Design review of the part built by this model. Coordinates are the model's own, in mm. Face numbers are marked on the shaded views. A direction names the side the tool comes from. Coordinates: 2 decimals unless noted, no trailing zeros. Write each loop counter-clockwise with the first axis right and the second up, starting at its lowest first coordinate (ties: lowest second). Pieces come first, ordered by that corner, then holes.
Q1. Take a section at B-B (z = 0.6). Give the boundary of the cut face in (x, y), and give its area (3 significant figures).
Q2. Mouldability with a two-part tool opening along X and no side actions: class the marked faces 4, 5 and 6 as pulls with the +X half, pulls with the -X half, needs draft (parallel to the pull), parting line crosses it, or undercut.
Q3. Insertion check: pin 1 (1.6 mm diameter, centred on y = -4.5, z = 2, fed in from -X); pin 2 (1.1 mm diameter, centred on x = 1.5, z = 1.5, fed in from -Y). Each pin has a flat end and moves straight along its axis. Give the tip position at first contact, or say it passes through.
Q4. For probe 1 along X at (y, z) = (-4.25, 0.8); probe 2 along X at (y, z) = (-5.25, 0.65); probe 3 along Y at (x, z) = (3.5, 0.75), list the stretches that pass through material, from the lowest coordinate up.
Q5. Take a section at D-D (y = -1). Give the boundary of the cut face in (x, z).
Q6. Take a section at A-A (y = -2.75). Give the boundary of the cut face in (x, z), and give its area (3 significant figures).
Q7. Machinability: for the marked faces 1, 2 and 3, which of the approach directions +Z, -Z, +X, -X, +Y, -Y give a long, thin tool a straight path to every point of the face, cutting with its end or side? Answer none if there is none.
Q8. Take a section at C-C (x = 6.25). Give the boundary of the cut face in (y, z).
```python
from build123d import *

# Parameters (mm, degrees)
EXTRUDE_1_DEPTH     = 3
SKETCH_4_R          = 1.5
EXTRUDE_3_DEPTH     = 1
SKETCH_8_W          = 1.758290516
SKETCH_8_H          = 4.288229266
SKETCH_8_W_2        = 1.505617074
SKETCH_8_H_2        = 4.786356908
CUT_EXTRUDE_3_DEPTH = 1


with BuildPart() as part:
    # 草图2 → 凸台-拉伸1 (new body)
    with BuildSketch(Plane.XY):
        with BuildLine():
            Line((5, 0), (2, 0))
            Line((2, 0), (0, -2))
            Line((0, -2), (0, -6))
            Line((0, -6), (1.9, -6))
            Line((1.9, -6), (1.9, -3.5))
            ThreePointArc((1.9, -3.5), (3.5, -1.9), (5.1, -3.5))
            Line((5.1, -3.5), (5.1, -6))
            Line((5.1, -6), (7, -6))
            Line((7, -6), (7, -2))
            Line((7, -2), (5, 0))
        make_face()
    extrude(amount=EXTRUDE_1_DEPTH)

    # 草图4 → 凸台-拉伸3 (add)
    with BuildSketch(Plane(origin=(0, 0, 0), x_dir=(1, 0, 0), z_dir=(0, 1, 0))):
        with Locations(Location((3.5, -1.5, 0), (0, 0, 270))):  # turned: the seam where the file's is
            Circle(SKETCH_4_R)
    extrude(amount=EXTRUDE_3_DEPTH)

    # 草图8 → 切除-拉伸3 (cut)
    with BuildSketch(Plane.XZ.offset(6)):
        with Locations((1.779145258, 1.583021274)):
            Rectangle(SKETCH_8_W, SKETCH_8_H)
        with Locations((5.347191463, 1.528876965)):
            Rectangle(SKETCH_8_W_2, SKETCH_8_H_2)
    extrude(amount=-CUT_EXTRUDE_3_DEPTH, mode=Mode.SUBTRACT)


solid = part.part
```
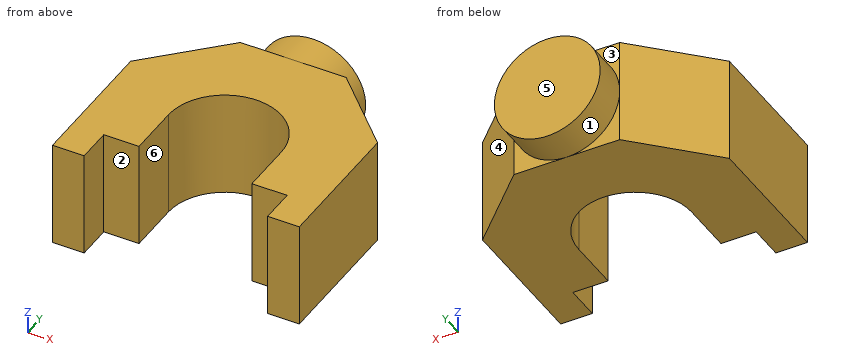
Response:
1. outline: (0, -6) - (0.9, -6) - (0.9, -5) - (1.9, -5) - (1.9, -3.5) arc R1.6 cw to (5.1, -3.5) - (5.1, -5) - (6.1, -5) - (6.1, -6) - (7, -6) - (7, -2) - (5, 0) - (4.7, 0) - (4.7, 1) - (2.3, 1) - (2.3, 0) - (2, 0) - (0, -2) - close
1. area: 26.4 mm2
2. face 4: pulls with the +X half
2. face 5: needs draft
2. face 6: undercut
3. pin 1: stops at x = 0
3. pin 2: stops at y = -5
4. probe 1: x = 0 to 1.9, 5.1 to 7
4. probe 2: x = 0 to 0.9, 6.1 to 7
4. probe 3: y = -1.9 to 1
5. outline: (1, 0) - (6, 0) - (6, 3) - (1, 3) - close
6. outline: (0, 0) - (2.09, 0) - (2.09, 3) - (0, 3) - close; (4.91, 0) - (7, 0) - (7, 3) - (4.91, 3) - close
6. area: 12.5 mm2
7. face 1: +Y
7. face 2: +Z, -Z, -Y
7. face 3: +Z, -X, +Y
8. outline: (-6, 0) - (-1.25, 0) - (-1.25, 3) - (-6, 3) - close
